Print and shaded views of the part. All mm, measured from the part's lowest x, y and z. Round coordinates to 2 decimals unless told otherwise and drop trailing zeros. Loops run counter-clockwise (first coordinate to the right, second up) from the corner with the lowest first, then second, coordinate; pieces in that order, holes last. Notation, with made-up numbers: (-21, 85.25) -> (34, 85.25) arc R20 cw to (34, 92.25) -> close; hole circle Ø7 at (87.5, 35). An arc over 180 degrees is marked (long way). Use a Markdown table: item, result.
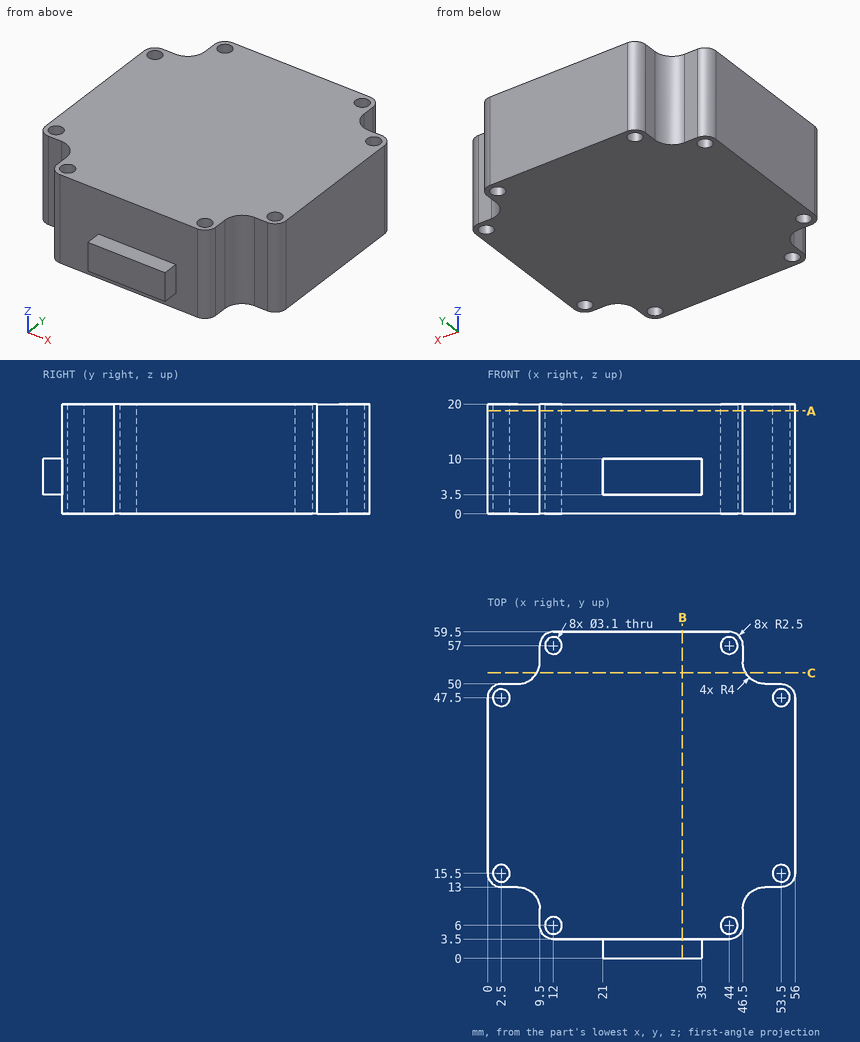
Q1. Flat gauge pins, fed straight in: pin 1 (2.5 mm diameter, centred on x = 4.5, z = 6, fed in from -Y); pin 2 (1.1 mm diameter, centred on x = 31.5, y = 2.5, fed in from -Z); pin 3 (1.5 mm diameter, centred on x = 4, z = 13.5, fed in from +Y); pin 4 (5 mm diameter, centred on x = 46.5, z = 10.5, fed in from +Y). Where does each tip first touch, or does it go through?
Results list:
| item | result |
|---|---|
| pin 1 | stops at y = 12.99 |
| pin 2 | stops at z = 3.5 |
| pin 3 | stops at y = 50 |
| pin 4 | stops at y = 59.5 |
Q2. Drill centre lines: L1, parallel to Y at x = 38, z = 16.5; L2, parallel to X at y = 9.5, z = 6; L3, parallel to Y at x = 46, z = 4.25. Where is each one in solid material? Low to high. Write a range as from..to.
Results list:
| item | result |
|---|---|
| L1 | y = 3.5..59.5 |
| L2 | x = 9.47..46.53 |
| L3 | y = 4.5..58.5 |
Q3. Band-saw the part on B-B, the plane x = 35.5. Give the cut face in (y, z).
Results list:
| item | result |
|---|---|
| outline | (0, 3.5) -> (3.5, 3.5) -> (3.5, 0) -> (59.5, 0) -> (59.5, 20) -> (3.5, 20) -> (3.5, 10) -> (0, 10) -> close |
Q4. Band-saw the part on C-C, the plane y = 52. Give the cut face in (x, z).
Results list:
| item | result |
|---|---|
| outline | (8.96, 0) -> (47.04, 0) -> (47.04, 20) -> (8.96, 20) -> close |
Q5. Band-saw the part on A-A, the plane z = 18.75. Give the number of separate pieces and of enclosed holes in the cut face, plus the area to 3 significant figures.
Results list:
| item | result |
|---|---|
| separate pieces | 1 |
| enclosed holes | 8 |
| area | 2,720 mm² |
